Check sheet for the modelled part. Datum: model origin and axes. Units: mm. Face numbers are marked on the shaded views. A direction names the side the tool comes from. Give positions to 0.01 mm unless a question says otherwise; leave off trailing zeros. Write each loop counter-clockwise with the first axis right and the second up, starting at its lowest first coordinate (ties: lowest second). Pieces come first, ordered by that corner, then holes. Notation, with made-up numbers: M 29.25,8.25 L 82.25,8.25 A21 cw 82.25,26.25 Z; hole C -13.5,49 d2. An arc over 180 degrees is marked long. Write item = value, one per line. Start each with the question number.
1) Cross-section at A-A, the plane y = 4.5. Record the cut outline in (x, z), plus the area to 3 significant figures.
2) Cross-section at B-B, the plane z = 0. Record the cut outline in (x, y).
3) Access from +Z, -Z, +X, -X, +Y, -Y to the whole of each face (thin tool, end or side, straight path). Record for the marked faces 1, 2 and 3.
4) Mould release check, pull along Z, two halves, no side actions. Record for the marked faces 4, 5 and 6: released by +Z, released by -Z, zero draft, split by the parting line, or undercut.
5) Cross-section at C-C, the plane z = 11. Give the number of separate pieces and of enclosed holes in the cut face, plus the area to 3 significant figures.
6) Scan lines: line 1 along X through (y, z) = (1.1, 11); line 2 along X through (y, z) = (5.5, 0); line 3 along Z through (x, y) = (0, 2). Record each from-to range of solid material in increasing order. Write a range as [from, to].
7) Go/stop test with flat-tipped pins: pin 1 (3 mm diameter, centred on x = -19.05, z = 11, fed in from +Y); pin 2 (6 mm diameter, centred on x = -4.5, y = 6, fed in from -Z); pin 3 (0.8 mm diameter, centred on y = 3, z = 18, fed in from +X). Record where each tip stops, or that it passes through.
```python
from build123d import *

# Parameters (mm, degrees)
SKETCH_2_R                  = 1.25
EXTRUDE_1491_DEPTH          = 3
FILLET_2_R                  = 3
FILLET_1631_R               = 5
CUT_EXTRUDE_2422_REACH      = 36.187
CUT_EXTRUDE_2422_END_RADIUS = 19.5
FILLET_4_R                  = 0.5
FILLET_5_R                  = 1


with BuildPart() as part:
    # Эскиз1 → Повернуть1 (revolve)
    with BuildSketch(Plane.XY):
        Polygon((0, 16), (0, 18), (19.5, 18), (19.5, 0), (17.5, 0), (17.5, 16), align=None)
    revolve(axis=Axis((0, 16, 0), (0, 1, 0)))

    # Эскиз2 → Extrude 1491 (add)
    # profile 1 of 4: a face of its own
    with BuildSketch(Plane.XZ):
        with BuildLine():
            Line((15.246008724, -16.056438521), (13.207625443, -14.346031861))
            ThreePointArc((13.207625443, -14.346031861), (14.937866641, -12.534358389), (16.421563491, -10.515809646))
            Line((16.421563491, -10.515809646), (18.459946773, -12.226216305))
            ThreePointArc((18.459946773, -12.226216305), (18.768088856, -15.748296437), (15.246008724, -16.056438521))
        make_face()
        with Locations(Location((16.852977749, -14.141327413, 0), (0, 0, 270))):
            Circle(SKETCH_2_R, mode=Mode.SUBTRACT)
    # profile 2 of 4: a face of its own
    with BuildSketch(Plane.XZ):
        with BuildLine():
            Line((-18.459946773, -12.226216305), (-16.421563491, -10.515809646))
            ThreePointArc((-16.421563491, -10.515809646), (-14.937866641, -12.534358389), (-13.207625443, -14.346031861))
            Line((-13.207625443, -14.346031861), (-15.246008724, -16.056438521))
            ThreePointArc((-15.246008724, -16.056438521), (-18.768088856, -15.748296437), (-18.459946773, -12.226216305))
        make_face()
        with Locations(Location((-16.852977749, -14.141327413, 0), (0, 0, 90))):
            Circle(SKETCH_2_R, mode=Mode.SUBTRACT)
    # profile 3 of 4: a face of its own
    with BuildSketch(Plane.XZ):
        with BuildLine():
            Line((17.802558883, 13.165063509), (15.498134224, 11.834603312))
            ThreePointArc((15.498134224, 11.834603312), (16.887495374, 9.75), (17.998134224, 7.504476293))
            Line((17.998134224, 7.504476293), (20.302558883, 8.834936491))
            ThreePointArc((20.302558883, 8.834936491), (21.217622393, 12.25), (17.802558883, 13.165063509))
        make_face()
        with Locations(Location((19.052558883, 11, 0), (0, 0, 270))):
            Circle(SKETCH_2_R, mode=Mode.SUBTRACT)
    # profile 4 of 4: a face of its own
    with BuildSketch(Plane.XZ):
        with BuildLine():
            Line((-20.302558883, 8.834936491), (-17.998134224, 7.504476293))
            ThreePointArc((-17.998134224, 7.504476293), (-16.887495374, 9.75), (-15.498134224, 11.834603312))
            Line((-15.498134224, 11.834603312), (-17.802558883, 13.165063509))
            ThreePointArc((-17.802558883, 13.165063509), (-21.217622393, 12.25), (-20.302558883, 8.834936491))
        make_face()
        with Locations(Location((-19.052558883, 11, 0), (0, 0, 90))):
            Circle(SKETCH_2_R, mode=Mode.SUBTRACT)
    extrude(amount=-EXTRUDE_1491_DEPTH)

    # Скругление2
    fillet_2_edges = [part.edges().sort_by_distance(p)[0] for p in [
        (-17.5, 16, 0),
    ]]
    fillet(fillet_2_edges, radius=FILLET_2_R)

    # Fillet 1631
    # the kernel refuses this fillet: 5 mm, written as the material it adds along each edge
    with BuildSketch(Plane(origin=(15.498134224, 0, 11.834603312), x_dir=(-0.6748484545014423, 0, 0.7379563425142538), z_dir=(0, 1, 0)), Plane(origin=(16.421563491, 0, -10.515809646), x_dir=(0.46264036439110967, 0, 0.8865460468785934), z_dir=(0, 1, 0)), Plane(origin=(-13.207625443, 0, -14.346031861), x_dir=(0.7927407641766817, 0, -0.6095589231670477), z_dir=(0, 1, 0)), Plane(origin=(-17.998134224, 0, 7.504476293), x_dir=(-0.301664712250469, 0, -0.9534140765600442), z_dir=(0, 1, 0))) as fillet_1631_piece_1:
        with BuildLine():
            CenterArc((3.893371259, 4.980387232), FILLET_1631_R, 202.918064629, 62.005438268)
            Line((-0.711942111, 3.033315388), (-1.172473448, 2.838608203))
            ThreePointArc((-1.172473448, 2.838608203), (-1.061572462, 2.490694934), (-0.488256583, -0.107728867))
            Line((-0.488256583, -0.107728867), (0.044242855, -0.498038723))
            ThreePointArc((0.044242855, -0.498038723), (1.725471354, -0.423510203), (3.406699852, -0.498038723))
            Line((3.406699852, -0.498038723), (3.450942707, 0))
        make_face()
    extrude(amount=3)
    with BuildSketch(Plane(origin=(17.998134224, 0, 7.504476293), x_dir=(0.3016647122504697, 0, -0.953414076560044), z_dir=(0, 1, 0)), Plane(origin=(13.207625443, 0, -14.346031861), x_dir=(-0.7927407641766814, 0, -0.609558923167048), z_dir=(0, 1, 0)), Plane(origin=(-16.421563491, 0, -10.515809646), x_dir=(-0.46264036439110884, 0, 0.886546046878594), z_dir=(0, 1, 0)), Plane(origin=(-15.498134224, 0, 11.834603312), x_dir=(0.674848454501442, 0, 0.7379563425142541), z_dir=(0, 1, 0))) as fillet_1631_piece_2:
        with BuildLine():
            CenterArc((3.893371259, -4.980387232), FILLET_1631_R, 95.076497103, 62.005438268)
            Line((-0.711942111, -3.033315388), (-1.172473448, -2.838608203))
            ThreePointArc((-1.172473448, -2.838608203), (-1.061572462, -2.490694934), (-0.488256583, 0.107728867))
            Line((-0.488256583, 0.107728867), (0.044242855, 0.498038723))
            ThreePointArc((0.044242855, 0.498038723), (1.725471354, 0.423510203), (3.406699852, 0.498038723))
            Line((3.406699852, 0.498038723), (3.450942707, 0))
        make_face()
    extrude(amount=3)

    # Cut-Extrude 2422: up to this cylinder (the profile starts inside it)
    cut_extrude_2422_end = Plane(origin=(0, 3.790585, 0), z_dir=(0, -1, 0)) * Cylinder(CUT_EXTRUDE_2422_END_RADIUS, 112.374, mode=Mode.PRIVATE)
    # Эскиз4 → Cut-Extrude 2422 (cut, up to the surface)
    with BuildSketch(Plane.XY, mode=Mode.PRIVATE) as cut_extrude_2422_sk1:
        with BuildLine():
            Line((-3.2, 5), (-3.2, 0))
            Line((-3.2, 0), (3.2, 0))
            Line((3.2, 0), (3.2, 5))
            ThreePointArc((3.2, 5), (0, 8.2), (-3.2, 5))
        make_face()
    cut_extrude_2422_tool1 = extrude(cut_extrude_2422_sk1.sketch, amount=CUT_EXTRUDE_2422_REACH, mode=Mode.PRIVATE) & cut_extrude_2422_end
    add(cut_extrude_2422_tool1.solids().sort_by_distance((0, 3.790585, 0))[0], mode=Mode.SUBTRACT)

    # Скругление4
    fillet_4_edges = [part.edges().sort_by_distance(p)[0] for p in [
        (1e-09, 8.200000026, 19.49999998),
        (-3.2, 2.5, 19.235643998),
        (3.2, 2.5, 19.235643998),
        (-3.2, 2.5, 17.204941151),
        (-3e-09, 8.200000027, 17.499999979),
        (3.2, 2.5, 17.204941151),
    ]]
    fillet(fillet_4_edges, radius=FILLET_4_R)

    # Скругление5
    fillet_5_edges = [part.edges().sort_by_distance(p)[0] for p in [
        (-19.5, 18, 0),
    ]]
    fillet(fillet_5_edges, radius=FILLET_5_R)


solid = part.part
```
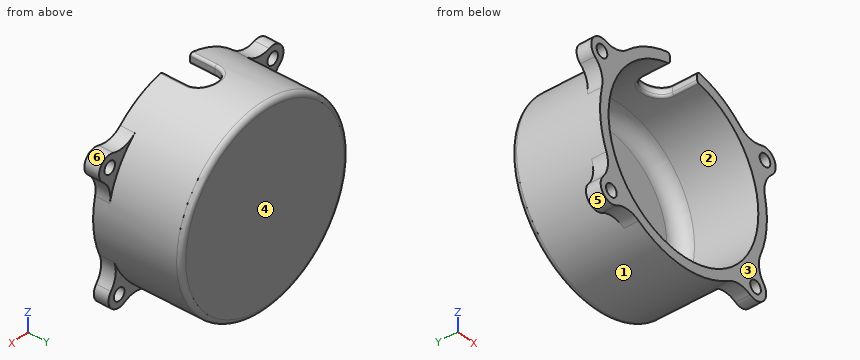
Reply:
q1.outline = M -3.8,19.13 A19.5 ccw long 3.8,19.13 A0.5 ccw 3.2,18.64 L 3.2,17.62 A0.5 ccw 3.6,17.13 A17.5 cw long -3.6,17.13 A0.5 ccw -3.2,17.62 L -3.2,18.64 A0.5 ccw Z
q1.area = 219 mm2
q2.outline = M -19.5,0 L -17.5,0 L -17.5,13 A3 cw -14.5,16 L 14.5,16 A3 cw 17.5,13 L 17.5,0 L 19.5,0 L 19.5,17 A1 ccw 18.5,18 L -18.5,18 A1 ccw -19.5,17 Z
q3.face_1 = +Y
q3.face_2 = -Y
q3.face_3 = +Z, -Z, +X, -X, -Y
q4.face_4 = zero draft
q4.face_5 = undercut
q4.face_6 = split by the parting line
q5.separate_pieces = 3
q5.enclosed_holes = 0
q5.area = 166 mm2
q6.line_1 = [-21.55, -20.3], [-17.8, -13.61], [13.61, 17.8], [20.3, 21.55]
q6.line_2 = [-19.5, -17.5], [17.5, 19.5]
q6.line_3 = [-19.5, -17.5]
q7.pin_1 = 3
q7.pin_2 = -19.44
q7.pin_3 = 8.4
